Geometry check sheet. Reference: the model listing, model coordinates, mm. Face numbers are marked on the shaded views. Give positions to 0.01 mm unless a question says otherwise; leave off trailing zeros. Order: outer loops, then holes, each group sorted by start corner. A loop starts at its lowest first (then second) coordinate and runs counter-clockwise, first axis right, second up. Notation, with made-up numbers: M 53,34 L 85,34 A27 cw 85,59 Z; hole C 20,87 d4. An arc over 180 degrees is marked long. Answer as CSV lines item,"result". Start each with the question number.
Autodesk Inventor part; units mm, degrees
ref_plane "YZ Plane" through (0, 0, 0) normal (1, 0, 0) x (0, 1, 0)
ref_plane "XZ Plane" through (0, 0, 0) normal (0, 1, 0) x (-1, 0, 0)
ref_plane "XY Plane" through (0, 0, 0) normal (0, 0, 1) x (1, 0, 0)
sketch "Sketch1" plane through (0, 0, 0) normal (0, 1, 0) x (-1, 0, 0)
  line L0 (0, -28) -> (0, 28)
  line L1 (16.8, 0) -> (-16.8, 0)
  line L2 (7, 15.25) -> (-7, 15.25)
  line L3 (-7, 15.25) -> (-7, -15.25)
  line L4 (-7, -15.25) -> (7, -15.25)
  line L5 (7, -15.25) -> (7, 15.25)
  line L6 (9, 17.25) -> (-9, 17.25)
  line L7 (-9, 17.25) -> (-9, -17.25)
  line L8 (-9, -17.25) -> (9, -17.25)
  line L9 (9, -17.25) -> (9, 17.25)
  line L10 (12, 20) -> (-12, 20)
  line L11 (-12, 20) -> (-12, -20)
  line L12 (-12, -20) -> (12, -20)
  line L13 (12, -20) -> (12, 20)
  point P0 (0, 0)
  dimension "d0" = 14
  dimension "d1" = 30.5
  dimension "d2" = 2
  dimension "d3" = 24
  dimension "d4" = 40
extrude "Extrusion1" add sketch "Sketch1" against normal blind 3 contours L8 L7 L1 L3 L4 L0 | L0 L4 L5 L1 L9 L8 | L7 L6 L0 L2 L3 L1 | L1 L5 L2 L0 L6 L9
extrude "Extrusion2" add sketch "Sketch1" along normal blind 2 contours L12 L11 L1 L7 L8 L0 | L0 L8 L9 L1 L13 L12 | L8 L7 L1 L3 L4 L0 | L0 L4 L5 L1 L9 L8 | L11 L10 L0 L6 L7 L1 | L1 L9 L6 L0 L10 L13 | L7 L6 L0 L2 L3 L1 | L1 L5 L2 L0 L6 L9
fillet "Fillet1" radius 1 4 edges at (-12, 2, 0) (0, 2, -20) (12, 2, 0) (0, 2, 20)
properties part number "Ramecek_3DPrint"
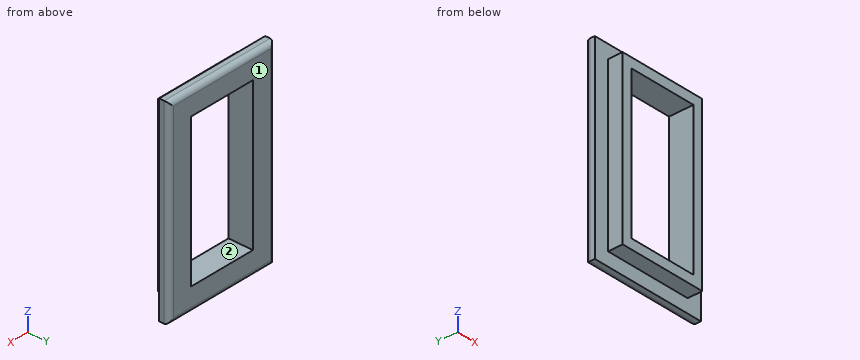
Item 1: Section check B-B on y = -1.4. Record the boundary of the cut face in (x, z).
Item 2: Section check D-D on y = 0.6. Record the boundary of the cut face in (x, z).
Item 3: Draft check along X on the marked faces 1 and 2. Enter one of: pulls with the +X half, pulls with the -X half, needs draft (parallel to the pull), parting line crosses it, or undercut.
Item 4: Depth check by flat-ended pin: pin 1 Ø1.5 at (x, y) = (-8.5, -1) entering from +Z; pin 2 Ø2.5 at (x, y) = (2, -1) entering from -Z; pin 3 Ø2.5 at (x, y) = (1, -1.5) entering from -Z; pin 4 Ø5 at (x, z) = (-0.5, 12) entering from +Y. Enter the tip coordinate at first touch or a pass-through.
Item 5: Section check C-C on z = -2. Record the boundary of the cut face in (x, y), then the cut area to 3 significant figures.
Item 6: Scan lines: line 1 along Z through (x, y) = (-2, -1.55); line 2 along X through (y, z) = (-2.6, 8); line 3 along X through (y, z) = (0.35, -8.5). Record each from-to range of solid material in increasing order.
Item 7: Section check A-A on x = -4.5. Record the boundary of the cut face in (y, z).
Numbers:
1,outline,"M -9,-17.25 L 9,-17.25 L 9,17.25 L -9,17.25 Z; hole M -7,-15.25 L 7,-15.25 L 7,15.25 L -7,15.25 Z"
2,outline,"M -12,-20 L 12,-20 L 12,20 L -12,20 Z; hole M -7,-15.25 L 7,-15.25 L 7,15.25 L -7,15.25 Z"
3,face 1,"needs draft"
3,face 2,"undercut"
4,pin 1,"z = 17.25"
4,pin 2,"z = -20"
4,pin 3,"z = -17.25"
4,pin 4,"through"
5,outline,"M -12,0 L -9,0 L -9,-3 L -7,-3 L -7,2 L -11,2 A1 ccw -12,1 Z; M 7,-3 L 9,-3 L 9,0 L 12,0 L 12,1 A1 ccw 11,2 L 7,2 Z"
5,area,"31.6 mm2"
6,line 1,"-17.25 to -15.25, 15.25 to 17.25"
6,line 2,"-9 to -7, 7 to 9"
6,line 3,"-12 to -7, 7 to 12"
7,outline,"M -3,-17.25 L 0,-17.25 L 0,-20 L 1,-20 A1 ccw 2,-19 L 2,-15.25 L -3,-15.25 Z; M -3,15.25 L 2,15.25 L 2,19 A1 ccw 1,20 L 0,20 L 0,17.25 L -3,17.25 Z"
